The listing builds one solid part. Answer for the finished solid, in the listing's coordinates (mm). Give positions to 0.01 mm unless a question says otherwise; leave off trailing zeros. Loops run counter-clockwise (first coordinate to the right, second up) from the corner with the lowest first, then second, coordinate; pieces in that order, holes last. Notation, with made-up numbers: (76, 5.5) - (128, 5.5) arc R20 ccw to (128, 29.5) - close; hole circle Ø7 at (-21, 26). An arc over 180 degrees is marked (long way). One line per item, written item: value. Start each with the question number.
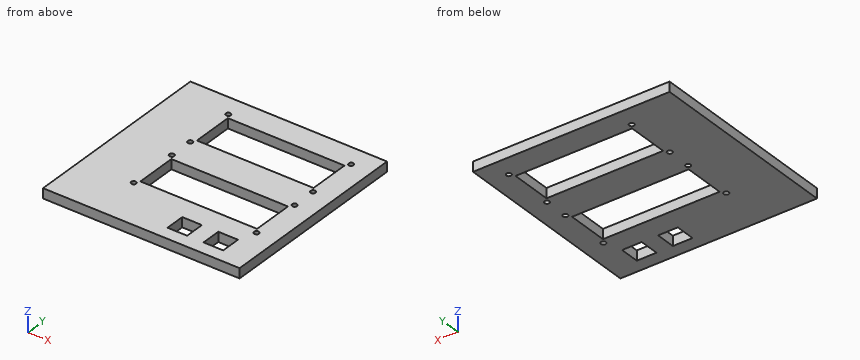
Autodesk Inventor part; units mm, degrees
ref_plane "YZ Plane" through (0, 0, 0) normal (1, 0, 0) x (0, 1, 0)
ref_plane "XZ Plane" through (0, 0, 0) normal (0, 1, 0) x (-1, 0, 0)
ref_plane "XY Plane" through (0, 0, 0) normal (0, 0, 1) x (1, 0, 0)
sketch "Sketch1" plane through (0, 0, 0) normal (0, 0, 1) x (1, 0, 0)
  line L0 (0, 0) -> (200, 0)
  line L1 (200, 0) -> (200, 120)
  line L2 (200, 120) -> (0, 120)
  line L3 (0, 120) -> (0, 0)
  line L4 (110, 110) -> (190, 110) construction
  line L5 (190, 110) -> (190, 74) construction
  line L6 (190, 74) -> (110, 74) construction
  line L7 (110, 74) -> (110, 110) construction
  line L8 (110, 64) -> (190, 64) construction
  line L9 (190, 64) -> (190, 28) construction
  line L10 (190, 28) -> (110, 28) construction
  line L11 (110, 28) -> (110, 64) construction
  circle A0 centre (112.5, 107.5) radius 1.5
  circle A1 centre (112.5, 61.5) radius 1.5
  circle A2 centre (187.5, 61.5) radius 1.5
  circle A3 centre (112.5, 30.5) radius 1.5
  circle A4 centre (187.5, 30.5) radius 1.5
  circle A5 centre (187.5, 107.5) radius 1.5
  circle A6 centre (112.5, 76.5) radius 1.5
  circle A7 centre (187.5, 76.5) radius 1.5
  line L12 (114.4, 104.6) -> (185.6, 104.6)
  line L13 (185.6, 104.6) -> (185.6, 79.4)
  line L14 (185.6, 79.4) -> (114.4, 79.4)
  line L15 (114.4, 79.4) -> (114.4, 104.6)
  line L16 (114.4, 58.6) -> (185.6, 58.6)
  line L17 (185.6, 58.6) -> (185.6, 33.4)
  line L18 (185.6, 33.4) -> (114.4, 33.4)
  line L19 (114.4, 33.4) -> (114.4, 58.6)
  dimension "d0" = 200
  dimension "d1" = 120
  dimension "d4" = 80
  dimension "d5" = 36
  dimension "d6" = 80
  dimension "d7" = 36
  dimension "d8" = 110
  dimension "d9" = 110
  dimension "d10" = 10
  dimension "d11" = 10
  dimension "d12" = 3
  dimension "d13" = 2.5
  dimension "d14" = 2.5
  dimension "d15" = 3
  dimension "d16" = 2.5
  dimension "d17" = 2.5
  dimension "d20" = 75
  dimension "d23" = 31
  dimension "d28" = 75
  dimension "d31" = 31
  dimension "d34" = 5.4
  dimension "d35" = 4.4
  dimension "d36" = 4.4
  dimension "d37" = 5.4
  dimension "d38" = 5.4
  dimension "d39" = 4.4
  dimension "d40" = 5.4
  dimension "d41" = 4.4
extrude "Extrusion1" add sketch "Sketch1" along normal blind 6
extrude "Extrusion2" cut sketch "Sketch1" along normal blind 75 contours A0 | A1 | A2 | A3 | A4 | A5 | A6 | A7 | L12 L13 L14 L15 | L16 L17 L18 L19
sketch "Sketch2" plane through (0, 0, 0) normal (0, 0, -1) x (-1, 0, 0)
  line L0 (-150, 8) -> (-162, 8)
  line L1 (-162, 8) -> (-162, 20)
  line L2 (-162, 20) -> (-150, 20)
  line L3 (-150, 20) -> (-150, 8)
  line L4 (-172, 8) -> (-184, 8)
  line L5 (-184, 8) -> (-184, 20)
  line L6 (-184, 20) -> (-172, 20)
  line L7 (-172, 20) -> (-172, 8)
  line L8 (0, 120) -> (0, 0)
  line L9 (-200, 120) -> (0, 120)
  point P0 (-150, 14)
  point P1 (-172, 14)
  dimension "d44" = 12
  dimension "d45" = 12
  dimension "d46" = 12
  dimension "d47" = 12
  dimension "d48" = 150
  dimension "d49" = 10
  dimension "d50" = 100
  dimension "d51" = 100
extrude "Extrusion3" cut sketch "Sketch2" against normal blind 6
sketch "Sketch3" plane through (0, 0, 6) normal (0, 0, 1) x (1, 0, 0)
  line L0 (0, 0) -> (200, 0)
  line L1 (0, 120) -> (80, 120)
  line L2 (80, 120) -> (80, 0)
  line L3 (80, 0) -> (0, 0)
  line L4 (0, 0) -> (0, 120)
  dimension "d54" = 80
extrude "Extrusion4" cut sketch "Sketch3" against normal blind 10
equation "\"d42\" = d28"
properties part number "lcd holder"
1. A cutting plane is placed at D-D (y = 61.5). Determine the outline of the cut face in (x, z).
2. A cutting plane is placed at C-C (x = 112.5). Determine the outline of the cut face in (y, z), plus the area to 3 significant figures.
3. A cutting plane is placed at B-B (z = 1.15). Give the number of separate pieces and of enclosed holes in the cut face, plus the area to 3 significant figures.
4. A cutting plane is placed at A-A (y = 96). Determine the outline of the cut face in (x, z), plus the area to 3 significant figures.
5. Find the intervals of material crossed by L1, parallel to X at y = 12, z = 3.2; L2, parallel to Y at x = 187.5, z = 1.45; L3, parallel to Y at x = 151, z = 3.7, in increasing order. Write a range as [from, to].
Results below:
1. outline: (80, 0) - (111, 0) - (111, 6) - (80, 6) - close; (114, 0) - (186, 0) - (186, 6) - (114, 6) - close; (189, 0) - (200, 0) - (200, 6) - (189, 6) - close
2. outline: (0, 0) - (29, 0) - (29, 6) - (0, 6) - close; (32, 0) - (60, 0) - (60, 6) - (32, 6) - close; (63, 0) - (75, 0) - (75, 6) - (63, 6) - close; (78, 0) - (106, 0) - (106, 6) - (78, 6) - close; (109, 0) - (120, 0) - (120, 6) - (109, 6) - close
2. area: 648 mm^2
3. separate pieces: 1
3. enclosed holes: 12
3. area: 10,500 mm^2
4. outline: (80, 0) - (114.4, 0) - (114.4, 6) - (80, 6) - close; (185.6, 0) - (200, 0) - (200, 6) - (185.6, 6) - close
4. area: 293 mm^2
5. L1: x = [80, 150], [162, 172], [184, 200]
5. L2: y = [0, 29], [32, 60], [63, 75], [78, 106], [109, 120]
5. L3: y = [0, 8], [20, 33.4], [58.6, 79.4], [104.6, 120]
